```python
from build123d import *

# Parameters (mm, degrees)
F1_DEPTH = 3.175
F2_R     = 1.5875
F3_DEPTH = 2.54


with BuildPart() as f1:
    # F0 (on Front) → F1 (new body)
    with BuildSketch(Plane.XZ):
        with BuildLine():
            Line((-51.3818325876, -3.121233064), (-4.5789436396, -11.8458125574))
            Line((-4.5789436396, -11.8458125574), (0.0033310249, -12.6999995632))
            ThreePointArc((0.0033310249, -12.6999995632), (12.6434077752, 1.1975975242), (-2.38125, 12.4747604561))
            Line((-2.38125, 12.4747604561), (-51.3953125, 3.118690114))
            ThreePointArc((-51.3953125, 3.118690114), (-53.9749925915, -0.006858838), (-51.3818325876, -3.121233064))
        make_face()
    extrude(amount=F1_DEPTH)

    # F2 (on face) → F3 (join)
    with BuildSketch(Plane.XZ.offset(3.175)):
        with Locations((-50.8, 0)):
            Circle(F2_R)
    extrude(amount=F3_DEPTH)


solid = f1.part
```
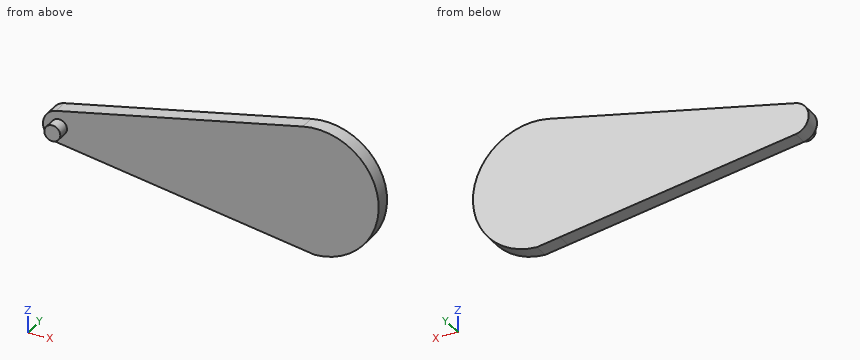
Part model, mm, in its own coordinate system. Round coordinates to 2 decimals unless told otherwise and drop trailing zeros. Loops run counter-clockwise (first coordinate to the right, second up) from the corner with the lowest first, then second, coordinate; pieces in that order, holes last. Notation, with made-up numbers: (75, 39) -> (83, 39) arc R30 cw to (83, 64) -> close; hole circle Ø8 at (25, -22.75). An arc over 180 degrees is marked (long way). Use one line per item in the form item = value. Start each with the question number.
Item 1: Band-saw the part on C-C (x = -50.8). List the corners of the cut face in (y, z) (1 decimal).
Item 2: Band-saw the part on D-D (z = 7.5). List the corners of the cut face in (x, y) (3 decimals).
Item 3: Drop flat-ended pins along their axis: pin 1 Ø12 at (x, z) = (-11.5, 5) entering from -Y (3 decimals); pin 2 Ø1 at (y, z) = (-2, 1.5) entering from +X. Give the stop position or say it passes through.
Item 4: Band-saw the part on A-A (z = 0). List the corners of the cut face in (x, y) (1 decimal).
Item 5: Band-saw the part on B-B (y = -1.35). List the corners of the cut face in (x, z) (3 decimals).
Item 6: Drill centre lines: line 1 along Y through (x, z) = (-8, -2.5) (3 decimals); line 2 along Z through (x, y) = (-4, -2.3); line 3 along Z through (x, y) = (-12, -2.6). Where is each one in solid material? Low to high.
Data:
q1.outline = (-5.7, -1.6) -> (-3.2, -1.6) -> (-3.2, -3.2) -> (0, -3.2) -> (0, 3.2) -> (-3.2, 3.2) -> (-3.2, 1.6) -> (-5.7, 1.6) -> close
q2.outline = (-28.443, -3.175) -> (10.249, -3.175) -> (10.249, 0) -> (-28.443, 0) -> close
q3.pin_1 = -3.175
q3.pin_2 = 12.66
q4.outline = (-54, -3.2) -> (-52.4, -3.2) -> (-52.4, -5.7) -> (-49.2, -5.7) -> (-49.2, -3.2) -> (12.7, -3.2) -> (12.7, 0) -> (-54, 0) -> close
q5.outline = (-51.395, 3.119) arc R3.175 ccw to (-51.382, -3.121) -> (0.003, -12.7) arc R12.7 ccw (long way) to (-2.381, 12.475) -> close
q6.line_1 = -3.175 to 0
q6.line_2 = -11.95 to 12.17
q6.line_3 = -10.46 to 10.64
